Design review of the part built by this model. Coordinates are the model's own, in mm. Face numbers are marked on the shaded views. A direction names the side the tool comes from. Coordinates: 2 decimals unless noted, no trailing zeros. Order: outer loops, then holes, each group sorted by start corner. A loop starts at its lowest first (then second) coordinate and runs counter-clockwise, first axis right, second up. Notation, with made-up numbers: M 87,-0.5 L 98,-0.5 A32 ccw 98,33.5 Z; hole C 28.25,-10 d9. An arc over 180 degrees is marked long. Answer as a JSON object with one key per item and string values.
from build123d import *

# Parameters (mm, degrees)
SKETCH1_R                = 0.5
SKETCH1_R_2              = 1.125
PCB_DEPTH                = 1.2
SKETCH2_R                = 3.15
SPEAKERS_DEPTH           = 5.5
SKETCH3_W                = 14
SKETCH3_H                = 14
LENS_MOUNT_DEPTH         = 10.5
LENS_MOUTING_HOLES_DEPTH = 5
SKETCH5_R                = 4.35
LENS_DEPTH               = 3.5


with BuildPart() as part:
    # Sketch1 → PCB (new body)
    with BuildSketch(Plane(origin=(0, 0, 0), x_dir=(1, 0, 0), z_dir=(0, 1, 0))):
        with BuildLine():
            Line((-36.8, -11), (-31.5, -11))
            Line((-31.5, -11), (-31.5, -9.45))
            ThreePointArc((-31.5, -9.45), (-30.75, -8.7), (-30, -9.45))
            Line((-30, -9.45), (-30, -11))
            Line((-30, -11), (-23.8, -11))
            Line((-23.8, -11), (-23.8, -10.35))
            ThreePointArc((-23.8, -10.35), (-22.95, -9.5), (-22.1, -10.35))
            Line((-22.1, -10.35), (-22.1, -11))
            Line((-22.1, -11), (29.7, -11))
            Line((29.7, -11), (29.7, -9.8))
            ThreePointArc((29.7, -9.8), (30.5, -9), (31.3, -9.8))
            Line((31.3, -9.8), (31.3, -11))
            Line((31.3, -11), (36.8, -11))
            Line((36.8, -11), (36.8, -6.5))
            ThreePointArc((36.8, -6.5), (37.092893219, -5.792893219), (37.8, -5.5))
            Line((37.8, -5.5), (39.8, -5.5))
            Line((39.8, -5.5), (39.8, 5.5))
            Line((39.8, 5.5), (37.8, 5.5))
            ThreePointArc((37.8, 5.5), (37.092893219, 5.792893219), (36.8, 6.5))
            Line((36.8, 6.5), (36.8, 11))
            Line((36.8, 11), (34.531625915, 11))
            Line((34.531625915, 11), (34.531625915, 10.4))
            ThreePointArc((34.531625915, 10.4), (32.881625915, 8.75), (31.231625915, 10.4))
            Line((31.231625915, 10.4), (31.231625915, 11))
            Line((31.231625915, 11), (29.016759255, 11))
            Line((29.016759255, 11), (29.016759255, 10.25))
            ThreePointArc((29.016759255, 10.25), (28.016759255, 9.25), (27.016759255, 10.25))
            Line((27.016759255, 10.25), (27.016759255, 11))
            Line((27.016759255, 11), (24.9, 11))
            Line((24.9, 11), (23.659748872, 8.106080701))
            ThreePointArc((23.659748872, 8.106080701), (23.291094851, 7.665158908), (22.740603842, 7.5))
            Line((22.740603842, 7.5), (-13.8, 7.5))
            Line((-13.8, 7.5), (-13.8, 3.194222302))
            ThreePointArc((-13.8, 3.194222302), (-15.5, 1.494222302), (-17.2, 3.194222302))
            Line((-17.2, 3.194222302), (-17.2, 7.5))
            Line((-17.2, 7.5), (-22.740603842, 7.5))
            ThreePointArc((-22.740603842, 7.5), (-23.291094851, 7.665158908), (-23.659748872, 8.106080701))
            Line((-23.659748872, 8.106080701), (-24.9, 11))
            Line((-24.9, 11), (-27.016759255, 11))
            Line((-27.016759255, 11), (-27.016759255, 10.25))
            ThreePointArc((-27.016759255, 10.25), (-28.016759255, 9.25), (-29.016759255, 10.25))
            Line((-29.016759255, 10.25), (-29.016759255, 11))
            Line((-29.016759255, 11), (-31.231625915, 11))
            Line((-31.231625915, 11), (-31.231625915, 10.4))
            ThreePointArc((-31.231625915, 10.4), (-32.881625915, 8.75), (-34.531625915, 10.4))
            Line((-34.531625915, 10.4), (-34.531625915, 11))
            Line((-34.531625915, 11), (-36.8, 11))
            Line((-36.8, 11), (-36.8, 6.5))
            ThreePointArc((-36.8, 6.5), (-37.092893219, 5.792893219), (-37.8, 5.5))
            Line((-37.8, 5.5), (-39.8, 5.5))
            Line((-39.8, 5.5), (-39.8, -5.5))
            Line((-39.8, -5.5), (-37.8, -5.5))
            ThreePointArc((-37.8, -5.5), (-37.092893219, -5.792893219), (-36.8, -6.5))
            Line((-36.8, -6.5), (-36.8, -11))
        make_face()
        with Locations((35.3, 9.5)):
            Circle(SKETCH1_R, mode=Mode.SUBTRACT)
        with Locations((-35.3, -9.75)):
            Circle(SKETCH1_R, mode=Mode.SUBTRACT)
        with Locations((-27.4, -9)):
            Circle(SKETCH1_R_2, mode=Mode.SUBTRACT)
        with Locations((35.3, -10)):
            Circle(SKETCH1_R, mode=Mode.SUBTRACT)
        with Locations((32.8, -10)):
            Circle(SKETCH1_R, mode=Mode.SUBTRACT)
    extrude(amount=PCB_DEPTH)

    # Sketch2 → speakers (add)
    with BuildSketch(Plane(origin=(0, 1.2, 0), x_dir=(1, 0, 0), z_dir=(0, 1, 0))):
        with Locations((-37.5, 0)):
            Circle(SKETCH2_R)
        with Locations((37.5, 0)):
            Circle(SKETCH2_R)
    extrude(amount=SPEAKERS_DEPTH)

    # Sketch3 → lens_mount (add)
    with BuildSketch(Plane(origin=(0, 1.2, 0), x_dir=(1, 0, 0), z_dir=(0, 1, 0))):
        with Locations((0.2, 0)):
            Rectangle(SKETCH3_W, SKETCH3_H)
    extrude(amount=LENS_MOUNT_DEPTH)

    # Sketch4 → lens_mouting_holes (add)
    with BuildSketch(Plane(origin=(0, 1.2, 0), x_dir=(1, 0, 0), z_dir=(0, 1, 0))):
        with BuildLine():
            Line((-8.55, 2.15), (8.95, 2.15))
            ThreePointArc((8.95, 2.15), (11.1, 0), (8.95, -2.15))
            Line((8.95, -2.15), (-8.55, -2.15))
            ThreePointArc((-8.55, -2.15), (-10.7, 0), (-8.55, 2.15))
        make_face()
    extrude(amount=LENS_MOUTING_HOLES_DEPTH)

    # Sketch5 → lens (add)
    with BuildSketch(Plane(origin=(0, 11.7, 0), x_dir=(1, 0, 0), z_dir=(0, 1, 0))):
        Circle(SKETCH5_R)
    extrude(amount=LENS_DEPTH)


solid = part.part
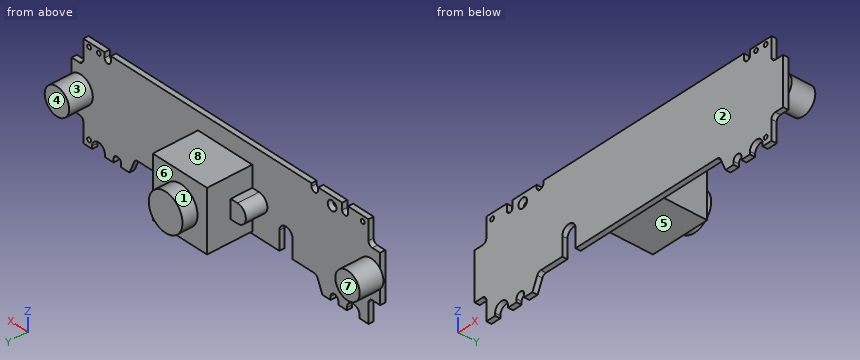
1) Mouldability with a two-part tool opening along X and no side actions: class the marked faces 1, 2 and 3 as released by +X, released by -X, zero draft, split by the parting line, or undercut.
Taken from the geometry:
{"face 1": "split by the parting line", "face 2": "zero draft", "face 3": "undercut"}
2) Insertion check: pin 1 Ø0.5 at (x, y) = (-7.5, 3) entering from -Z; pin 2 Ø3 at (x, y) = (5, 9.5) entering from +Z; pin 3 Ø1.3 at (y, z) = (0.5, 9) entering from +X; pin 4 Ø1 at (x, y) = (27, 2) entering from -Z. Each pin has a flat end and moves straight along its axis. Give the tip position at first contact, or say it passes through.
Taken from the geometry:
{"pin 1": "stops at z = -2.15", "pin 2": "stops at z = 7", "pin 3": "stops at x = 36.8", "pin 4": "passes through"}
3) Add section B-B (y = 13). State the section outline as (x, z) points.
Taken from the geometry:
{"outline": "C 0,0 d8.7"}
4) Add section D-D (x = -15.5). State the section outline as (y, z) points.
Taken from the geometry:
{"outline": "M 0,-1.49 L 1.2,-1.49 L 1.2,11 L 0,11 Z"}
5) To check wall thickness, follow L1, parallel to Z at x = 35.3, y = 0.5; L2, parallel to Z at x = -35.3, y = 0.3; L3, parallel to Z at x = 32.8, y = 0.5. State the ranges of each line that lie inside material, in increasing order.
Taken from the geometry:
{"L1": "z = -11 to -10, -9 to 9.5, 10.5 to 11", "L2": "z = -11 to 9.25, 10.25 to 11", "L3": "z = -8.75 to 9.5, 10.5 to 11"}
6) Add section C-C (z = 0.75). State the section outline as (x, y) points.
Taken from the geometry:
{"outline": "M -40.56,1.2 L -39.8,1.2 L -39.8,0 L 39.8,0 L 39.8,1.2 L 40.56,1.2 L 40.56,6.7 L 34.44,6.7 L 34.44,1.2 L 10.96,1.2 L 10.96,6.2 L 7.2,6.2 L 7.2,11.7 L 4.28,11.7 L 4.28,15.2 L -4.28,15.2 L -4.28,11.7 L -6.8,11.7 L -6.8,6.2 L -10.56,6.2 L -10.56,1.2 L -34.44,1.2 L -34.44,6.7 L -40.56,6.7 Z"}
7) Add section A-A (x = 0). State the section outline as (y, z) points, and give its area (3 significant figures).
Taken from the geometry:
{"outline": "M 0,-7.5 L 1.2,-7.5 L 1.2,-7 L 11.7,-7 L 11.7,-4.35 L 15.2,-4.35 L 15.2,4.35 L 11.7,4.35 L 11.7,7 L 1.2,7 L 1.2,11 L 0,11 Z", "area": "200 mm2"}
8) Tool access review of the marked faces 4, 5, 6, 7 and 8: name each direction out of +Z, -Z, +X, -X, +Y, -Y from which nothing blocks a thin tool from reaching the whole face with its end or side.
Taken from the geometry:
{"face 4": "+Z, -Z, +X, +Y", "face 5": "-Z, +X, -X, +Y", "face 6": "+Y", "face 7": "+Z, -Z, -X, +Y", "face 8": "+Z, +X, -X, +Y"}
